```python
from build123d import *

# Parameters (mm, degrees)
R_VOLUTION1_ANGLE       = 180
ESQUISSE2_R             = 9
ENL_V_MAT_EXTRU_1_DEPTH = 31


with BuildPart() as part:
    # Esquisse1 → Révolution1 (revolve)
    with BuildSketch(Plane.XY):
        with BuildLine():
            Line((0, 17), (0, 75))
            Line((0, 75), (2, 75))
            ThreePointArc((2, 75), (15, 62), (28, 75))
            Line((28, 75), (30, 75))
            Line((30, 75), (30, 17))
            Line((30, 17), (0, 17))
        make_face()
    revolve(axis=Axis((0, 0, 0), (1, 0, 0)), revolution_arc=R_VOLUTION1_ANGLE)

    # Esquisse2 → Enlèv. mat.-Extru.1 (cut, through all)
    with BuildSketch(Plane.ZY):
        with Locations((37, 0)):
            Circle(ESQUISSE2_R)
        with Locations((13, -34.641016151)):
            Circle(ESQUISSE2_R)
        with Locations((13, 34.641016151)):
            Circle(ESQUISSE2_R)
    extrude(amount=-ENL_V_MAT_EXTRU_1_DEPTH, mode=Mode.SUBTRACT)


solid = part.part
```
The listing builds one solid part. Answer for the finished solid, in the listing's coordinates (mm). Coordinates: 2 decimals unless noted, no trailing zeros. Write each loop counter-clockwise with the first axis right and the second up, starting at its lowest first coordinate (ties: lowest second). Pieces come first, ordered by that corner, then holes. Notation, with made-up numbers: (77.25, -33) - (101.25, -33) arc R16 cw to (101.25, -16) - close; hole circle Ø6 at (46.5, -26). An arc over 180 degrees is marked (long way). Return JSON: item names as keys, results as strings. Group by question number.
Q1. The part is cut by section C-C on z = 13. State how many separate pieces and enclosed holes the cut face has, and give its area (3 significant figures).
Q2. The part is cut by section A-A on y = 0. Write down the section's boundary in (x, z).
Q3. Flat-ended cylindrical pins translate along their axes: pin 1 Ø3 at (x, z) = (5.5, 26.5) entering from -Y; pin 2 Ø1.5 at (x, z) = (20, 27) entering from +Y; pin 3 Ø4 at (x, z) = (7.5, 55.5) entering from -Y; pin 4 Ø11 at (y, z) = (34.64, 13) entering from +X. Find the tip coordinate at first contact, or state that the pin passes through.
Q4. The part is cut by section B-B on x = 12.5. Write down the section's boundary in (y, z).
Q5. For a pull along Y with two mould halves and no side action, classify faces 1 (the cylindrical face through (15, 0, 17)), 2 (the cylindrical face through (1.01, 1.65, 74.98)), 3 (the flat face through (30, -1, 46.4)), 4 (the cylindrical face through (14.79, -43.427, 11.049)) as +Y half, -Y half, draft (parallel to the pull), parting line (faces both ways), or undercut.
Q6. The part is cut by section D-D on x = 23.5. Write down the section's boundary in (y, z), and give its area (3 significant figures).
Q7. Find the intervals of material crossed by line 1 along Y through (x, z) = (17.75, 13); line 2 along Y through (x, z) = (17, 19); line 3 along Y through (x, z) = (12.75, 13), in increasing order. Write a range as [from, to].
Evaluation:
{
 "1": {"separate pieces": "4", "enclosed holes": "0", "area": "2,150 mm2"},
 "2": {"outline": "(0, 17) - (30, 17) - (30, 28) - (0, 28) - close; (0, 46) - (30, 46) - (30, 75) - (28, 75) arc R13 cw to (2, 75) - (0, 75) - close"},
 "3": {"pin 1": "stops at y = -62.78", "pin 2": "stops at y = 57.43", "pin 3": "stops at y = -37.02", "pin 4": "passes through"},
 "4": {"outline": "(-62.24, 0) - (-17, 0) arc R17 cw to (17, 0) - (62.24, 0) arc R62.24 ccw to start; hole circle Ø18 at (-34.64, 13); hole circle Ø18 at (0, 37); hole circle Ø18 at (34.64, 13)"},
 "5": {"face 1": "undercut", "face 2": "parting line", "face 3": "draft", "face 4": "undercut"},
 "6": {"outline": "(-65.16, 0) - (-17, 0) arc R17 cw to (17, 0) - (65.16, 0) arc R65.16 ccw to start; hole circle Ø18 at (-34.64, 13); hole circle Ø18 at (0, 37); hole circle Ø18 at (34.64, 13)", "area": "5,450 mm2"},
 "7": {"line 1": "y = [-60.92, -43.64], [-25.64, -10.95], [10.95, 25.64], [43.64, 60.92]", "line 2": "y = [-59.18, -41.35], [-27.93, 27.93], [41.35, 59.18]", "line 3": "y = [-60.82, -43.64], [-25.64, -10.95], [10.95, 25.64], [43.64, 60.82]"}
}
